Read the model definition and answer for the solid it produces. Units are mm, in the model's axes. A direction names the side the tool comes from. Coordinates: 2 decimals unless noted, no trailing zeros. Write each loop counter-clockwise with the first axis right and the second up, starting at its lowest first coordinate (ties: lowest second). Pieces come first, ordered by that corner, then holes. Notation, with made-up numbers: (48, -28) -> (94, -28) arc R16 ccw to (94, -20) -> close; hole circle Ø7 at (76, 25.5). An arc over 180 degrees is marked (long way). Answer as a JSON object with one key per item and string values. Group by question number.
(1) For a pull along X with two mould halves and no side action, classify faces 3 (the face through (51, 7, 18)), 4 (the face through (100, 3, 17)), 5 (the face through (83.4, 2.03, 17.43)) as +X half, -X half, draft (parallel to the pull), parting line (faces both ways), or undercut.
(2) Find section B-B (x = 85). Give the vertices of the cut face in (y, z), then the cut area to 3 significant figures.
(3) Find section A-A (z = 17.5). Give the vertices of the cut face in (x, y), then the cut area to 3 significant figures.
(4) Which of the six approach directions +Z, -Z, +X, -X, +Y, -Y give full straight-line access (tool end or side, diameter ignored) to faces 1 (the face through (82.5, 5.5, 17.4)), 2 (the face through (0, 3, 18))?
(5) Straight lines are drawn through the part: L1, parallel to Z at x = 85, y = 5; L2, parallel to X at y = 2.95, z = 17.5; L3, parallel to X at y = 5.65, z = 17.5. For each, find the intervals that lie inside material, in ascending order.
Autodesk Inventor part; units mm, degrees
ref_plane "YZ Plane" through (0, 0, 0) normal (1, 0, 0) x (0, 1, 0)
ref_plane "XZ Plane" through (0, 0, 0) normal (0, 1, 0) x (-1, 0, 0)
ref_plane "XY Plane" through (0, 0, 0) normal (0, 0, 1) x (1, 0, 0)
sketch "Sketch1" plane through (0, 0, 0) normal (0, 1, 0) x (-1, 0, 0)
  line L0 (0, 0) -> (-100, 0)
  line L1 (-100, 0) -> (-100, 35)
  line L2 (-100, 35) -> (0, 35)
  line L3 (0, 35) -> (0, 0)
  dimension "d0" = 100
  dimension "d1" = 35
extrude "Extrusion1" add sketch "Sketch1" along normal blind 7
sketch "Sketch2" plane through (0, 7, 0) normal (0, 1, 0) x (1, 0, 0)
  line L0 (0, 0) -> (0, -35)
  line L1 (100, -35) -> (100, 0)
  circle A0 centre (85, -17.5) radius 1.5
  line L2 (0, -35) -> (100, -35)
  line L3 (50, -35) -> (50, 0)
  line L4 (100, 0) -> (0, 0)
  circle A1 centre (85, -17.5) radius 2.5
  point P0 (0, -17.5)
  dimension "d6" = 3
  dimension "d8" = 5
extrude "Extrusion2" cut sketch "Sketch2" against normal blind 3 contours A0 | A1
sketch "Sketch3" plane through (85, 4, 17.5) normal (0, 1, 0) x (1, 0, 0)
  circle A0 centre (0, 0) radius 1.6
  point P0 (-85, 17.5)
  dimension "d11" = 3.2
extrude "Extrusion3" cut sketch "Sketch3" against normal blind 4
sketch "Sketch4" plane through (0, 7, 0) normal (0, 1, 0) x (1, 0, 0)
  line L0 (100, -35) -> (100, 0)
  line L1 (0, 0) -> (0, -35)
  point P0 (0, -17.5)
  dimension "d14" = 100
  dimension "d15" = 35
properties part number "piano di carico"
Results below:
{
 "1": {"face 3": "draft", "face 4": "+X half", "face 5": "undercut"},
 "2": {"outline": "(0, 0) -> (7, 0) -> (7, 15) -> (4, 15) -> (4, 15.9) -> (0, 15.9) -> close; (0, 19.1) -> (4, 19.1) -> (4, 20) -> (7, 20) -> (7, 35) -> (0, 35) -> close", "area": "217 mm2"},
 "3": {"outline": "(0, 0) -> (83.4, 0) -> (83.4, 4) -> (82.5, 4) -> (82.5, 7) -> (0, 7) -> close; (86.6, 0) -> (100, 0) -> (100, 7) -> (87.5, 7) -> (87.5, 4) -> (86.6, 4) -> close", "area": "672 mm2"},
 "4": {"face 1": "+Y", "face 2": "+Z, -Z, -X, +Y, -Y"},
 "5": {"L1": "z = 0 to 15, 20 to 35", "L2": "x = 0 to 83.4, 86.6 to 100", "L3": "x = 0 to 82.5, 87.5 to 100"}
}
